Geometry check sheet. Reference: drawing and pictorial views, mm from the part's lowest x, y, z. Coordinates: 2 decimals unless noted, no trailing zeros. Loops run counter-clockwise (first coordinate to the right, second up) from the corner with the lowest first, then second, coordinate; pieces in that order, holes last.
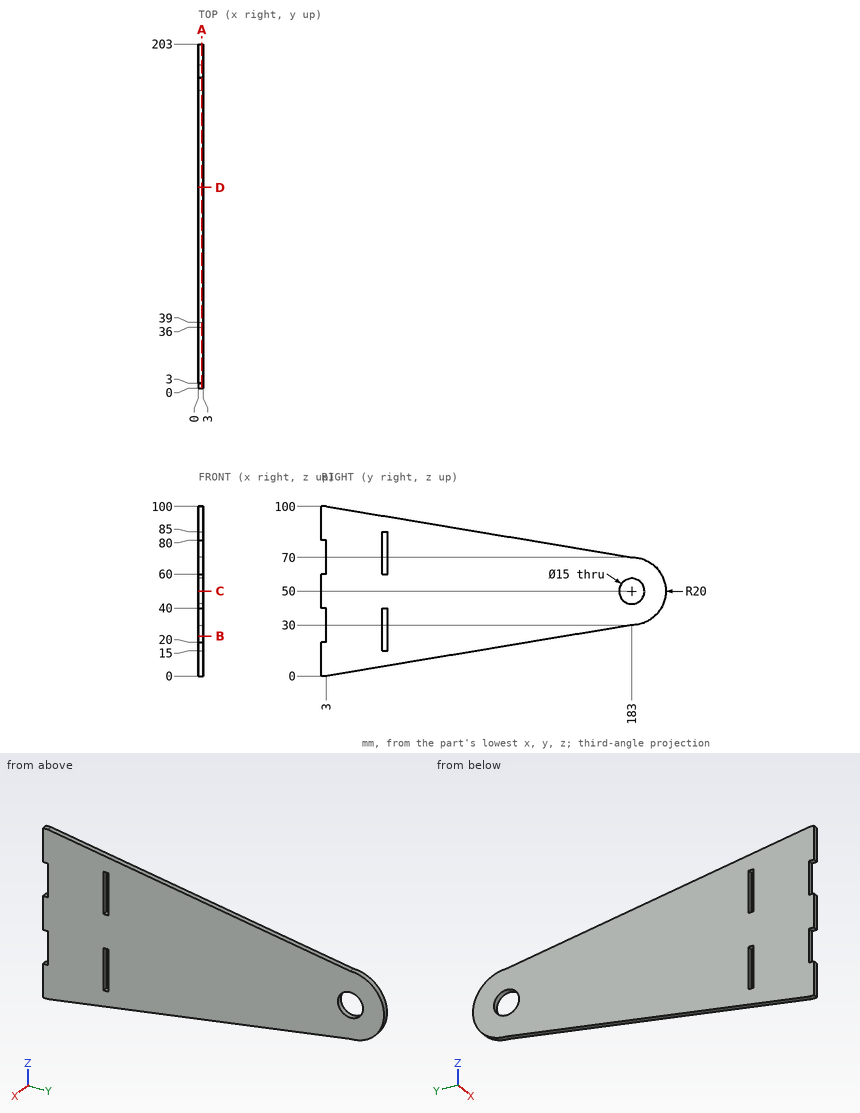
1) Section check D-D on y = 118.5. Record the cut outline in (x, z).
Data:
outline: (0, 19.25) - (3, 19.25) - (3, 80.75) - (0, 80.75) - close
2) Section check A-A on x = 2.05. Record the cut outline in (y, z), and give its area (3 significant figures).
Data:
outline: (0, 0) - (3, 0) - (183, 30) arc R20 ccw to (183, 70) - (3, 100) - (0, 100) - (0, 80) - (3, 80) - (3, 60) - (0, 60) - (0, 40) - (3, 40) - (3, 20) - (0, 20) - close; hole (36, 15) - (39, 15) - (39, 40) - (36, 40) - close; hole (36, 60) - (39, 60) - (39, 85) - (36, 85) - close; hole circle Ø15 at (183, 50)
area: 13,100 mm2
3) Material ranges on probe 1 along Z at (x, y) = (1.55, 183.5); probe 2 along Y at (x, z) = (1.55, 50); probe 3 along Z at (x, y) = (2.5, 178), recorded low to high.
Data:
probe 1: z = 30.01 to 42.52, 57.48 to 69.99
probe 2: y = 0 to 175.5, 190.5 to 203
probe 3: z = 29.17 to 44.41, 55.59 to 70.83
4) Depth check by flat-ended pin: pin 1 (1.5 mm diameter, centred on x = 1.5, y = 37, fed in from -Z); pin 2 (1 mm diameter, centred on x = 2, y = 58.5, fed in from -Z); pin 3 (0.9 mm diameter, centred on x = 1, z = 24.5, fed in from -Y). Enter the tip coordinate at first touch or a pass-through.
Data:
pin 1: stops at z = 5.54
pin 2: stops at z = 9.17
pin 3: stops at y = 3
5) Section check B-B on z = 23.5. Record the cut outline in (x, y).
Data:
outline: (0, 3) - (3, 3) - (3, 36) - (0, 36) - close; (0, 39) - (3, 39) - (3, 144) - (0, 144) - close
6) Section check C-C on z = 50. Record the cut outline in (x, y), and give its area (3 significant figures).
Data:
outline: (0, 0) - (3, 0) - (3, 175.5) - (0, 175.5) - close; (0, 190.5) - (3, 190.5) - (3, 203) - (0, 203) - close
area: 564 mm2
